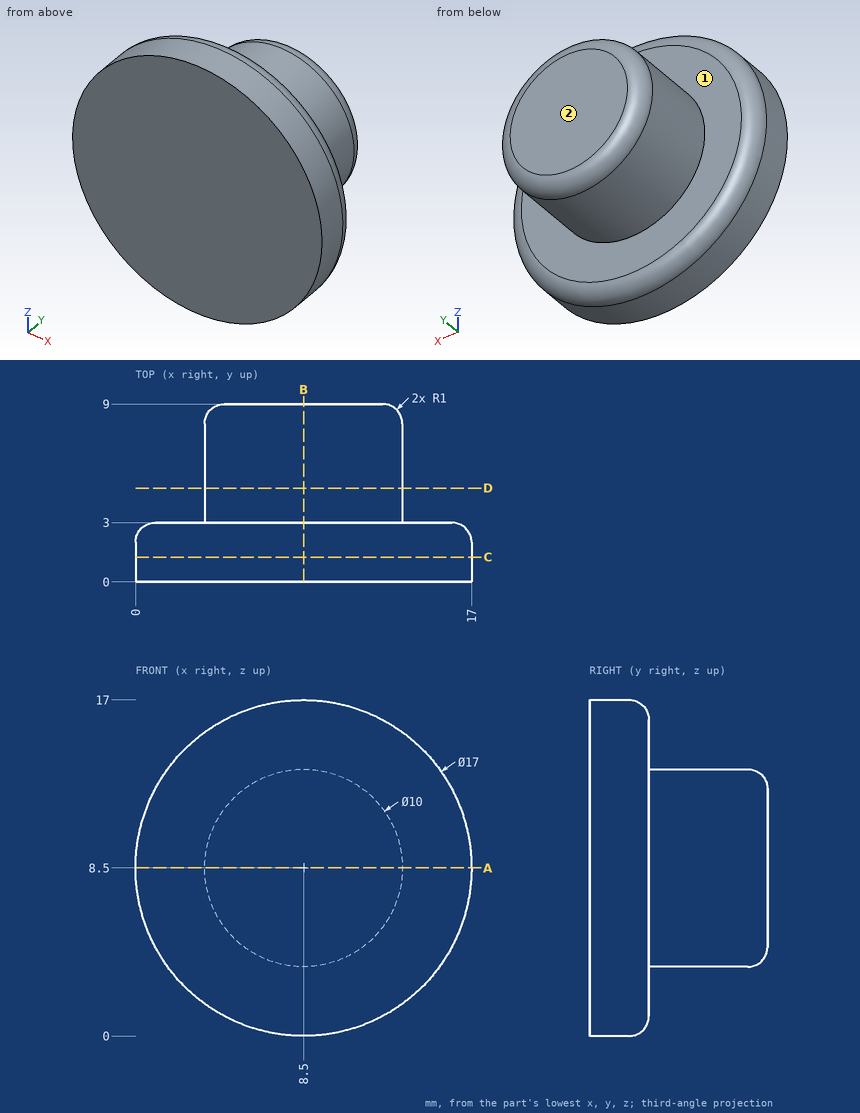
Can you work these out from the drawing? Everything is in mm from the part's minimum corner. A direction names the side the tool comes from. Coordinates: 2 decimals unless noted, no trailing zeros. Order: outer loops, then holes, each group sorted by start corner. A loop starts at its lowest first (then second) coordinate and runs counter-clockwise, first axis right, second up. Notation, with made-up numbers: M 32.5,-0.75 L 48.5,-0.75 A21 cw 48.5,37.25 Z; hole C 72,35 d4. An arc over 180 degrees is marked long. Answer as CSV lines item,"result". Start each with the question number.
1. For pin 1 (1.5 mm diameter, centred on y = 1, z = 7.5, fed in from -X); pin 2 (1 mm diameter, centred on y = 7.5, z = 11.5, fed in from -X); pin 3 (3 mm diameter, centred on x = 8, y = 6.5, fed in from -Z), each with a flat end and sliding along its axis, tell me the tip position at first contact or that it passes through.
2. I want a section at A-A, the plane z = 8.5. Write out the boundary of the cut face in (x, y).
3. I want a section at D-D, the plane y = 4.75. Write out the boundary of the cut face in (x, z).
4. I want a section at C-C, the plane y = 1.25. Write out the boundary of the cut face in (x, z).
5. I want a section at B-B, the plane x = 8.5. Write out the boundary of the cut face in (y, z).
6. I need wall thicknesses on line 1 (Y direction, x = 5.75, z = 13.25); line 2 (X direction, y = 5.75, z = 5.5); line 3 (Z direction, x = 11.75, y = 1.25). Which ranges of each line are inside material? Lowest first, please. Write a range as [from, to].
7. On a 3-axis mill with a long thin cutter (end or side, diameter ignored), from which of +Z, -Z, +X, -X, +Y, -Y can I reach the whole of each face in a straight line? I mean the marked faces 1 and 2. Say none if no direction works.
Recorded:
1,pin 1,"stops at x = 0"
1,pin 2,"stops at x = 4.17"
1,pin 3,"stops at z = 3.5"
2,outline,"M 0,0 L 17,0 L 17,2 A1 ccw 16,3 L 13.5,3 L 13.5,8 A1 ccw 12.5,9 L 4.5,9 A1 ccw 3.5,8 L 3.5,3 L 1,3 A1 ccw 0,2 Z"
3,outline,"C 8.5,8.5 d10"
4,outline,"C 8.5,8.5 d17"
5,outline,"M 0,0 L 2,0 A1 ccw 3,1 L 3,3.5 L 8,3.5 A1 ccw 9,4.5 L 9,12.5 A1 ccw 8,13.5 L 3,13.5 L 3,16 A1 ccw 2,17 L 0,17 Z"
6,line 1,"y = [0, 3]"
6,line 2,"x = [4.5, 12.5]"
6,line 3,"z = [0.65, 16.35]"
7,face 1,"+Y"
7,face 2,"+Z, -Z, +X, -X, +Y"
